from build123d import *

# Parameters (mm, degrees)
SKETCH_1_W        = 100
SKETCH_1_H        = 100
EXTRUDE_1_DEPTH   = 2
CHAMFER_1_SIZE    = 2
HOLE_WIZARD_M81_D = 9


with BuildPart() as part:
    # Эскиз1 → Бобышка-Вытянуть1 (new body)
    with BuildSketch(Plane.XY):
        Rectangle(SKETCH_1_W, SKETCH_1_H)
    extrude(amount=EXTRUDE_1_DEPTH)

    # Фаска1
    chamfer_1_edges = [part.edges().sort_by_distance(p)[0] for p in [
        (50, -50, 1),
        (-50, -50, 1),
        (-50, 50, 1),
        (50, 50, 1),
    ]]
    chamfer(chamfer_1_edges, length=CHAMFER_1_SIZE)

    # Отверстие с зазором M81 (through all)
    with Locations(Plane.XY.offset(2)):
        with Locations((-25, 25), (25, 25), (-25, -25), (25, -25)):
            Hole(HOLE_WIZARD_M81_D / 2)


solid = part.part
Geometry check sheet. Reference: the model listing, model coordinates, mm. Round coordinates to 2 decimals unless told otherwise and drop trailing zeros. Loops run counter-clockwise (first coordinate to the right, second up) from the corner with the lowest first, then second, coordinate; pieces in that order, holes last. Notation, with made-up numbers: (40, 18) -> (51, 18) arc R17 cw to (51, 39) -> close; hole circle Ø11 at (40.5, 18.5). An arc over 180 degrees is marked (long way). Answer as a JSON object with one key per item and string values. Group by question number.
Item 1: Thickness scan on line 1 along Y through (x, z) = (25, 0.4); line 2 along X through (y, z) = (27, 1). Record the ranges inside material, lowest first.
Item 2: Release check for a two-part mould opening along X. For faces 1 (the face through (-1, 1, 2)), 2 (the face through (28.32, 28.04, 0.99)), 3 (the face through (-21.68, 28.04, 0.99)) record: pulls with the +X half, pulls with the -X half, needs draft (parallel to the pull), parting line crosses it, or undercut.
Item 3: Cross-section at A-A, the plane y = 25. Record the cut outline in (x, z), plus the area to 3 significant figures.
Item 4: Depth check by flat-ended pin: pin 1 Ø7 at (x, y) = (-25, -25) entering from +Z. Enter the tip coordinate at first touch or a pass-through.
Item 5: Cross-section at C-C, the plane z = 1.4. Record the cut outline in (x, y).
Determined:
{
 "1": {"line 1": "y = -50 to -29.5, -20.5 to 20.5, 29.5 to 50", "line 2": "x = -50 to -29.03, -20.97 to 20.97, 29.03 to 50"},
 "2": {"face 1": "needs draft", "face 2": "undercut", "face 3": "undercut"},
 "3": {"outline": "(-50, 0) -> (-29.5, 0) -> (-29.5, 2) -> (-50, 2) -> close; (-20.5, 0) -> (20.5, 0) -> (20.5, 2) -> (-20.5, 2) -> close; (29.5, 0) -> (50, 0) -> (50, 2) -> (29.5, 2) -> close", "area": "164 mm²"},
 "4": {"pin 1": "passes through"},
 "5": {"outline": "(-50, -48) -> (-48, -50) -> (48, -50) -> (50, -48) -> (50, 48) -> (48, 50) -> (-48, 50) -> (-50, 48) -> close; hole circle Ø9 at (-25, -25); hole circle Ø9 at (-25, 25); hole circle Ø9 at (25, -25); hole circle Ø9 at (25, 25)"}
}
